```python
from build123d import *

# Parameters (mm, degrees)
SKETCH_1_R          = 20
SKETCH_1_R_2        = 15
EXTRUDE_1_DEPTH     = 3
SKETCH_2_R          = 2.5
CUT_EXTRUDE_1_DEPTH = 92.262525064
SKETCH_3_R          = 5
CUT_EXTRUDE_2_DEPTH = 10


with BuildPart() as part:
    # 草图1 → 凸台-拉伸1 (new body)
    with BuildSketch(Plane(origin=(0, 0, 0), x_dir=(1, 0, 0), z_dir=(0, 1, 0))):
        Circle(SKETCH_1_R)
        with BuildLine():
            ThreePointArc((20, 0), (8.309115435, -18.192267607), (-13.095860068, -15.116165158))
            Line((-13.095860068, -15.116165158), (39.675579632, -60.834598551))
            ThreePointArc((39.675579632, -60.834598551), (38.890872965, -38.890872965), (60.834598551, -39.675579632))
            Line((60.834598551, -39.675579632), (15.116165158, 13.095860068))
            ThreePointArc((15.116165158, 13.095860068), (18.73930766, 6.98844392), (20, 0))
        make_face()
        with Locations((49.497474683, -49.497474683)):
            Circle(SKETCH_1_R_2)
    extrude(amount=EXTRUDE_1_DEPTH)

    # 草图2 → 切除-拉伸1 (cut, through all)
    with BuildSketch(Plane(origin=(0, 3, 0), x_dir=(1, 0, 0), z_dir=(0, 1, 0))):
        with Locations(Location((0, 0, 0), (0, 0, 270))):
            Circle(SKETCH_2_R)
    extrude(amount=-CUT_EXTRUDE_1_DEPTH, mode=Mode.SUBTRACT)

    # 草图3 → 切除-拉伸2 (cut)
    with BuildSketch(Plane(origin=(0, 3, 0), x_dir=(1, 0, 0), z_dir=(0, 1, 0))):
        with Locations(Location((0, 0, 0), (0, 0, 270))):
            Circle(SKETCH_3_R)
    extrude(amount=-CUT_EXTRUDE_2_DEPTH, mode=Mode.SUBTRACT)


solid = part.part
```
For this review, take the finished solid that the model builds, in its own axes (mm). Round coordinates to 2 decimals unless told otherwise and drop trailing zeros. Order: outer loops, then holes, each group sorted by start corner. A loop starts at its lowest first (then second) coordinate and runs counter-clockwise, first axis right, second up.
Q1. We need section B-B, the plane x = 3. Give the boundary of the cut face in (y, z).
Findings below:
outline: (0, -19.77) - (3, -19.77) - (3, -4) - (0, -4) - close; (0, 4) - (3, 4) - (3, 29.06) - (0, 29.06) - close
Q2. We need section D-D, the plane z = -11.5. Give the boundary of the cut face in (x, y).
Findings below:
outline: (-16.36, 0) - (16.5, 0) - (16.5, 3) - (-16.36, 3) - close
Q3. Insertion check: P1, Ø9, axis at x = 0, z = 0, coming from the -Y side; P2, Ø1.5, axis at y = 0.5, z = 51.5, coming from the -X side. Each pin has a flat end and moves straight along its axis. Give the tip position at first contact, or say it passes through.
Findings below:
P1: passes through
P2: stops at x = 28.04
Q4. Wall thickness on line 1 (X direction, y = 2.35, z = 3.5); line 2 (X direction, y = 1.4, z = 0.5); line 3 (Z direction, x = -7, y = 0.55) (3 decimals): over which ranges is each line inside the solid? List them lowest first.
Findings below:
line 1: x = -19.69 to -3.57, 3.57 to 29.49
line 2: x = -19.99 to -4.97, 4.97 to 26.89
line 3: z = -18.735 to 20.397
Q5. We need section A-A, the plane z = 0. Give the boundary of the cut face in (x, y), plus the area to 3 significant figures.
Findings below:
outline: (-20, 0) - (-5, 0) - (-5, 3) - (-20, 3) - close; (5, 0) - (26.46, 0) - (26.46, 3) - (5, 3) - close
area: 109 mm2
Q6. We need section C-C, the plane y = 2.5. Give the boundary of the cut face in (x, z).
Findings below:
outline: (-13.1, 15.12) arc R20 ccw (long way) to (15.12, -13.1) - (60.83, 39.68) arc R15 ccw to (39.68, 60.83) - close; hole circle Ø10 at (0, 0)
Q7. Mouldability with a two-part tool opening along Z and no side actions: class faces 1 (the flat face through (22, 3, 22)), 2 (the cylindrical face through (-4.88, 1.52, -1.08)), 3 (the cylindrical face through (59.879, 1.479, 60.324)) as pulls with the +Z half, pulls with the -Z half, needs draft (parallel to the pull), parting line crosses it, or undercut.
Findings below:
face 1: needs draft
face 2: undercut
face 3: parting line crosses it
